```python
from build123d import *

# Parameters (mm, degrees)
SKETCH2_R           = 3.25
CUT_EXTRUDE1_DEPTH  = 61.713794973
BOSS_EXTRUDE1_START = -14
SKETCH4_R           = 37.5
SKETCH4_R_2         = 30
BOSS_EXTRUDE1_DEPTH = 14
CHAMFER1_SIZE       = 1
CIRPATTERN1_COUNT   = 3
CIRPATTERN1_ANGLE   = 60
M6_TAPPED_HOLE1_D   = 5


with BuildPart() as part:
    # Sketch1 → Revolve1 (revolve)
    with BuildSketch(Plane(origin=(0, 0, 0), x_dir=(1, 0, 0), z_dir=(0, 1, 0)), mode=Mode.PRIVATE) as revolve1_sk:
        Polygon((0, 20), (24, 20), (24, 30), (43.43, 30), (43.43, 15), (0, 15), align=None)
    revolve(revolve1_sk.sketch.rotate(Axis((0, 0, 0), (1, 0, 0)), 180), axis=Axis((0, 0, 0), (1, 0, 0)))

    # Sketch2 → Cut-Extrude1 (cut, through all)
    with BuildSketch(Plane(origin=(43.43, 0, 0), x_dir=(0, 0, -1), z_dir=(1, 0, 0))):
        with Locations((0, 25)):
            Circle(SKETCH2_R)
        with Locations((25, 0)):
            Circle(SKETCH2_R)
        with Locations((-25, 0)):
            Circle(SKETCH2_R)
        with Locations((0, -25)):
            Circle(SKETCH2_R)
    cut_extrude1 = extrude(amount=-CUT_EXTRUDE1_DEPTH, mode=Mode.SUBTRACT)

    # Sketch4 → Boss-Extrude1 (add)
    with BuildSketch(Plane.ZY.offset(-24).offset(BOSS_EXTRUDE1_START)):
        Circle(SKETCH4_R)
        Circle(SKETCH4_R_2, mode=Mode.SUBTRACT)
    extrude(amount=BOSS_EXTRUDE1_DEPTH)

    # Chamfer1
    chamfer1_edges = [part.edges().sort_by_distance(p)[0] for p in [
        (38, 0, -30),
        (38, 0, -37.5),
        (24, 0, -37.5),
        (0, 0, -15),
        (43.43, 0, -15),
        (43.43, 0, -30),
        (24, 0, -20),
        (0, 0, -20),
    ]]
    chamfer(chamfer1_edges, length=CHAMFER1_SIZE)

    # CirPattern1: Cut-Extrude1 ×3 about axis
    cirpattern1_axis = Axis((0, 0, 0), (-1, 0, 0))
    for i in range(1, CIRPATTERN1_COUNT):
        add(cut_extrude1.rotate(cirpattern1_axis, i * CIRPATTERN1_ANGLE / (CIRPATTERN1_COUNT - 1)), mode=Mode.SUBTRACT)

    # M6 Tapped Hole1 (through all)
    with Locations(Plane.ZY.offset(-24)):
        with Locations((-8.411618966, 31.392589354), (31.392589354, 8.411618966), (8.411618966, -31.392589354), (-31.392589354, -8.411618966)):
            Hole(M6_TAPPED_HOLE1_D / 2)


solid = part.part
```
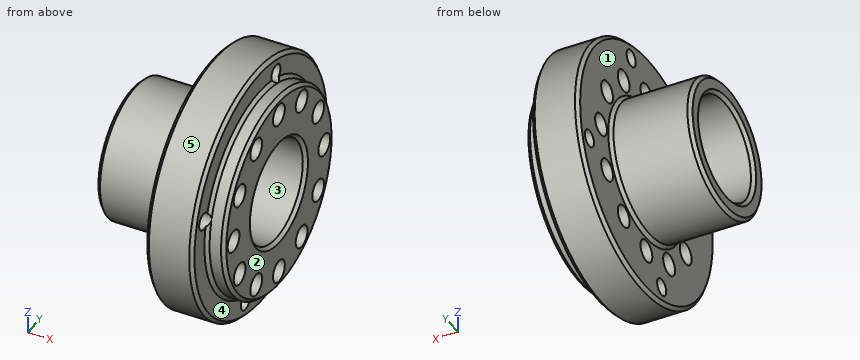
Verification items for the finished model (mm, model axes). Face numbers are marked on the shaded views. A direction names the side the tool comes from. Coordinates: 2 decimals unless noted, no trailing zeros. Write each loop counter-clockwise with the first axis right and the second up, starting at its lowest first coordinate (ties: lowest second). Pieces come first, ordered by that corner, then holes. Notation, with made-up numbers: M 45.25,-24.5 L 76.25,-24.5 A23 cw 76.25,12.5 Z; hole C 16.5,50.25 d1. An arc over 180 degrees is marked long. One line per item, written item: value.
Item 1: Access from +Z, -Z, +X, -X, +Y, -Y to the whole of each face (thin tool, end or side, straight path). Record for the marked faces 1 and 2.
Check sheet entries:
face 1: -X
face 2: +Z, -Z, +X, +Y, -Y
Item 2: Section check A-A, the plane z = 0. State how many separate pieces and enclosed holes the cut face has, plus the area to 3 significant figures.
Check sheet entries:
separate pieces: 4
enclosed holes: 0
area: 776 mm^2
Item 3: Gauge pin test, flat ends, axial feed: pin 1 Ø6.5 at (y, z) = (-31.39, 8.41) entering from -X; pin 2 Ø12 at (x, y) = (24.5, 29) entering from -Z; pin 3 Ø6 at (y, z) = (-21.65, 12.5) entering from -X; pin 4 Ø12 at (y, z) = (-9, 5) entering from -X. Record the tip position at first contact, or that the pin passes through.
Check sheet entries:
pin 1: stops at x = 24
pin 2: stops at z = -29.6
pin 3: passes through
pin 4: stops at x = 0
Item 4: Mould release check, pull along Z, two halves, no side actions. Record for the marked faces 3, 4 and 5: pulls with the +Z half, pulls with the -Z half, needs draft (parallel to the pull), parting line crosses it, or undercut.
Check sheet entries:
face 3: undercut
face 4: needs draft
face 5: parting line crosses it
Item 5: Section check D-D, the plane x = 5. Record the boundary of the cut face in (y, z).
Check sheet entries:
outline: C 0,0 d40; hole C 0,0 d30
Item 6: Scan lines: line 1 along Y through (x, z) = (32.5, 0); line 2 along Y through (x, z) = (29, -11); line 3 along Z through (x, y) = (39, -23.5). Record each from-to range of solid material in increasing order.
Check sheet entries:
line 1: y = -37.5 to -28.25, -21.75 to -15, 15 to 21.75, 28.25 to 37.5
line 2: y = -35.85 to -24.53, -18.77 to -10.2, 10.2 to 18.77, 24.53 to 35.85
line 3: z = -18.65 to -15.17, -9.83 to -2.88, 2.88 to 9.83, 15.17 to 18.65
